Could you check a few things on this model? Use its own coordinates, in mm. Coordinates: 2 decimals unless noted, no trailing zeros. Write each loop counter-clockwise with the first axis right and the second up, starting at its lowest first coordinate (ties: lowest second). Pieces come first, ordered by that corner, then holes.
Item 1: I want a section at D-D on x = -3. Please give me the cut outline in (y, z).
Item 2: I want a section at A-A on x = -0.25. Please give me the cut outline in (y, z).
Item 3: If I drill on probe 1 along X at (y, z) = (1.85, -3.5); probe 2 along Z at (x, y) = (0, 2.1); probe 3 along X at (y, z) = (1.95, 6.5), over which ranges is the centre line in solid material (lowest first)?
Item 4: I want a section at C-C on z = 8. Please give me the cut outline in (x, y).
Item 5: For P1, Ø1.5, axis at y = 1, z = -2, coming from the +X side, with a flat end and sliding along its axis, tell me the tip position at first contact or that it passes through.
Item 6: Thinking about a two-plate mould opening in Z: for faces 1 (the flat face through (3.99, 1, 2)), 2 (the cylindrical face through (-3.53, 1.52, -14.66)), 3 (the cylindrical face through (-0.13, 1.52, 7.5)), 4 (the cylindrical face through (-0.13, 1.52, 1.5)), which applies, +Z half, -Z half, draft (parallel to the pull), parting line (faces both ways), or undercut?
Item 7: I want a section at B-B on y = 0.55. State how many separate pieces and enclosed holes the cut face has, then the cut area to 3 significant figures.
Autodesk Inventor part; units mm, degrees
ref_plane "YZ Plane" through (0, 0, 0) normal (1, 0, 0) x (0, 1, 0)
ref_plane "XZ Plane" through (0, 0, 0) normal (0, 1, 0) x (-1, 0, 0)
ref_plane "XY Plane" through (0, 0, 0) normal (0, 0, 1) x (1, 0, 0)
sketch "Sketch1" plane through (0, 0, 0) normal (0, 1, 0) x (-1, 0, 0)
  line L0 (4.0096, 14.964) -> (-3.9904, 14.964)
  line L1 (-3.9904, 14.964) -> (-3.9904, -12.0894)
  line L2 (4.0096, -15.036) -> (4.0096, 14.964)
  line L3 (4.0096, 14.964) -> (-4.018, -14.9952) construction
  line L4 (-3.9904, 14.964) -> (4.0096, -15.036) construction
  line L5 (4.0096, -15.036) -> (-6.0407, -16.8081)
  line L6 (-3.9904, -12.0894) -> (-6.4901, -13.5325)
  line L7 (-6.4901, -13.5325) -> (-6.0407, -16.8081)
  point P0 (0, 0)
  dimension "d5" = 30
  dimension "d6" = 8
  dimension "d7" = 7.812
  dimension "d8" = 120
  dimension "d9" = 100
  dimension "d10" = 3.2756
  dimension "d11" = 27.0534
  dimension "d12" = 45
extrude "Extrusion1" add sketch "Sketch1" along normal blind 3
fillet "Fillet1" radius 2 4 edges at (-4.0096, 1.5, -15.036) (6.0407, 1.5, -16.8081) (6.4901, 1.5, -13.5325) (3.9904, 1.5, -12.0894)
sketch "Sketch2" plane through (0, 3, 0) normal (0, 1, 0) x (1, 0, 0)
  circle A0 centre (-0.0096, -6.964) radius 0.55
  line L0 (-4.0096, -14.964) -> (3.9904, -14.964)
  line L1 (-4.0096, 13.3578) -> (-4.0096, -14.964)
  circle A1 centre (-0.0096, -0.964) radius 0.55
  point P0 (0, 0)
  dimension "d16" = 8
  dimension "d17" = 1.1
  dimension "d18" = 4
  dimension "d19" = 14
  dimension "d20" = 4
  dimension "d21" = 1.1
extrude "Extrusion2" cut sketch "Sketch2" against normal blind 3
properties part number "remoteswitchtouch"
Response values:
1. outline: (0, -15.1) - (3, -15.1) - (3, 14.96) - (0, 14.96) - close
2. outline: (0, -15.7) - (3, -15.7) - (3, 0.47) - (0, 0.47) - close; (0, 1.46) - (3, 1.46) - (3, 6.47) - (0, 6.47) - close; (0, 7.46) - (3, 7.46) - (3, 14.96) - (0, 14.96) - close
3. probe 1: x = -4.01 to 3.99
3. probe 2: z = -15.74 to 0.41, 1.51 to 6.41, 7.51 to 14.96
3. probe 3: x = -4.01 to -0.3, 0.29 to 3.99
4. outline: (-4.01, 0) - (3.99, 0) - (3.99, 3) - (-4.01, 3) - close
5. P1: stops at x = 3.99
6. face 1: draft
6. face 2: -Z half
6. face 3: undercut
6. face 4: undercut
7. separate pieces: 1
7. enclosed holes: 2
7. area: 250 mm2
